Can you work these out from the model? Positions are in its coordinate system, mm. Face numbers are marked on the shaded views. Round coordinates to 2 decimals unless told otherwise and drop trailing zeros. Order: outer loops, then holes, each group sorted by start corner. A loop starts at its lowest first (then second) coordinate and runs counter-clockwise, first axis right, second up.
Q1. If we section it at A-A (z = 38): Please give me the cut outline in (x, y) (1 decimal).
Q2. If I drill on line 1 (X direction, y = 0.75, z = 38) (1 decimal); line 2 (X direction, y = 2, z = 41.5); line 3 (Z direction, x = -10, y = 2), over which ranges is the centre line in solid material (lowest first)?
Q3. If we section it at B-B (y = -2.5): Please give me the cut outline in (x, z), plus the area to 3 significant figures.
Q4. We'd pull the mould along X, two halves only. Please class the marked faces 1 and 2: pulls with the +X half, pulls with the -X half, needs draft (parallel to the pull), parting line crosses it, or undercut.
Q5. If we section it at C-C (x = 30): Please give me the cut outline in (y, z) (3 decimals).
Q6. Will these pins go through, and if not, where does the flat tip stop? P1, Ø3.5, axis at x = -30.5, y = 2.5, coming from the +Z side; P2, Ø2.5, axis at x = 24.5, y = 1.5, coming from the +Z side.
Q7. If we section it at D-D (z = -5.5): Please give me the cut outline in (x, y) (1 decimal), plus the area to 3 significant figures.
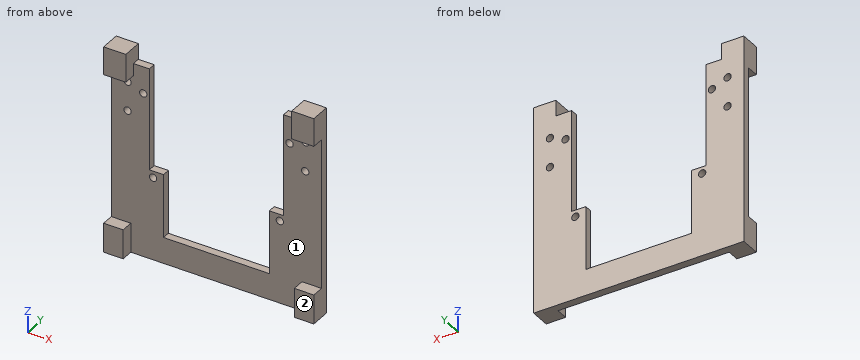
from build123d import *

# Parameters (mm, degrees)
BOSS_EXTRUDE4_DEPTH  = 3.175
M3_CLEARANCE_HOLE3_D = 3
M3_CLEARANCE_HOLE1_D = 3.1
M3_CLEARANCE_HOLE4_D = 2.95
M3_CLEARANCE_HOLE2_D = 3.1
CUT_EXTRUDE1_DEPTH   = 121.250075364
BOSS_EXTRUDE6_DEPTH  = 3.175
CUT_EXTRUDE3_DEPTH   = 121.250075364
SKETCH25_R           = 1.5
CUT_EXTRUDE4_DEPTH   = 121.250075364
SKETCH26_W           = 55
SKETCH26_H           = 60
CUT_EXTRUDE5_DEPTH   = 10
SKETCH27_OUTSIDE_W   = 217.324
SKETCH27_OUTSIDE_H   = 197.151
SKETCH27_OUTSIDE_W_2 = 86.188981544
SKETCH27_OUTSIDE_H_2 = 85
CUT_EXTRUDE6_DEPTH   = 10
SKETCH32_W           = 68
SKETCH32_H           = 11.5
CUT_EXTRUDE9_DEPTH   = 78.908304199
SKETCH33_W           = 9.094490772
SKETCH33_H           = 11.5
SKETCH33_W_2         = 8
SKETCH33_H_2         = 12
BOSS_EXTRUDE7_DEPTH  = 5
SKETCH34_W           = 6.5
SKETCH34_H           = 3.175
BOSS_EXTRUDE8_DEPTH  = 5
SKETCH35_R           = 1.5
CUT_EXTRUDE10_DEPTH  = 79.271667052
SKETCH38_W           = 18
SKETCH38_H           = 3.175
BOSS_EXTRUDE10_DEPTH = 5.8
SKETCH39_W           = 18
SKETCH39_H           = 3.175
BOSS_EXTRUDE11_DEPTH = 5.8
SKETCH37_R           = 1.5
CUT_EXTRUDE14_DEPTH  = 79.271667052
SKETCH40_W           = 43.4
SKETCH40_H           = 8
CUT_EXTRUDE15_DEPTH  = 79.271667052


with BuildPart() as part:
    # Sketch1 → Boss-Extrude4 (new body)
    with BuildSketch(Plane(origin=(0, 0, 0), x_dir=(1, 0, 0), z_dir=(0, 1, 0))):
        with BuildLine():
            Line((-62.799553621, 32.496136604), (-73.969425011, 32.691107434))
            Line((-73.969425011, 32.691107434), (-77.053684287, 35.88495141))
            ThreePointArc((-77.053684287, 35.88495141), (-84.36642289, 10.358894189), (-83.446216027, -16.178041625))
            Line((-83.446216027, -16.178041625), (-79.680911643, -13.825218315))
            Line((-79.680911643, -13.825218315), (-69.484649137, -16.179210996))
            Line((-69.484649137, -16.179210996), (-43.094490772, -58.412292655))
            Line((-43.094490772, -58.412292655), (-43.094490772, -64.826600275))
            Line((-43.094490772, -64.826600275), (-34, -64.826600275))
            Line((-34, -64.826600275), (-34, -58.55))
            Line((-34, -58.55), (34, -58.55))
            Line((34, -58.55), (34, -64.826600275))
            Line((34, -64.826600275), (43.094490772, -64.826600275))
            Line((43.094490772, -64.826600275), (43.094490772, -58.412292655))
            Line((43.094490772, -58.412292655), (69.484649137, -16.179210996))
            Line((69.484649137, -16.179210996), (79.680911643, -13.825218315))
            Line((79.680911643, -13.825218315), (83.446216027, -16.178041625))
            ThreePointArc((83.446216027, -16.178041625), (84.36642289, 10.358894189), (77.053684287, 35.88495141))
            Line((77.053684287, 35.88495141), (73.969425011, 32.691107434))
            Line((73.969425011, 32.691107434), (62.799553621, 32.496136604))
            Line((62.799553621, 32.496136604), (30.284668021, 63.895396642))
            Line((30.284668021, 63.895396642), (30.089697191, 75.065268032))
            Line((30.089697191, 75.065268032), (33.173956467, 78.259112008))
            ThreePointArc((33.173956467, 78.259112008), (0, 85), (-33.173956467, 78.259112008))
            Line((-33.173956467, 78.259112008), (-30.089697191, 75.065268032))
            Line((-30.089697191, 75.065268032), (-30.284668021, 63.895396642))
            Line((-30.284668021, 63.895396642), (-62.799553621, 32.496136604))
        make_face()
    extrude(amount=BOSS_EXTRUDE4_DEPTH)

    # M3 Clearance Hole3 (through all)
    with Locations(Plane(origin=(0, 0, 0), x_dir=(-1, 0, 0), z_dir=(0, -1, 0))):
        with Locations((36.415, -50), (36.415, -38), (-36.415, -50), (-36.415, -38)):
            Hole(M3_CLEARANCE_HOLE3_D / 2)

    # M3 Clearance Hole1 (through all)
    with Locations(Plane(origin=(0, 3.175, 0), x_dir=(1, 0, 0), z_dir=(0, 1, 0))):
        with Locations((-78.542321426, -8.49139241), (78.542321426, -8.49139241), (74.155025063, 27.240269049), (-74.155025063, 27.240269049)):
            Hole(M3_CLEARANCE_HOLE1_D / 2)

    # M3 Clearance Hole4 (through all)
    with Locations(Plane(origin=(0, 0, 0), x_dir=(-1, 0, 0), z_dir=(0, -1, 0))):
        with Locations((-67.099301622, -15.278865202), (-50.141885166, -42.416404279), (-61.062544382, 30.698137949), (-38.043670771, 52.927205804), (50.141885166, -42.416404279), (67.099301622, -15.278865202), (38.043670771, 52.927205804), (61.062544382, 30.698137949)):
            Hole(M3_CLEARANCE_HOLE4_D / 2)

    # M3 Clearance Hole2 (through all)
    with Locations(Plane(origin=(0, 3.175, 0), x_dir=(1, 0, 0), z_dir=(0, 1, 0))):
        with Locations((27, 76.497766718), (-27, 76.497766718)):
            Hole(M3_CLEARANCE_HOLE2_D / 2)

    # Sketch20 → Cut-Extrude1 (cut, through all)
    with BuildSketch(Plane(origin=(0, 3.175, 0), x_dir=(1, 0, 0), z_dir=(0, 1, 0))):
        with BuildLine():
            Line((-14.64850035, 45.5), (-14.64850035, 40.5))
            ThreePointArc((-14.64850035, 40.5), (-16.14850035, 39), (-17.64850035, 40.5))
            Line((-17.64850035, 40.5), (-17.64850035, 45.5))
            ThreePointArc((-17.64850035, 45.5), (-16.14850035, 47), (-14.64850035, 45.5))
        make_face()
        with BuildLine():
            Line((14.64850035, 45.5), (14.64850035, 40.5))
            ThreePointArc((14.64850035, 40.5), (16.14850035, 39), (17.64850035, 40.5))
            Line((17.64850035, 40.5), (17.64850035, 45.5))
            ThreePointArc((17.64850035, 45.5), (16.14850035, 47), (14.64850035, 45.5))
        make_face()
    extrude(amount=-CUT_EXTRUDE1_DEPTH, mode=Mode.SUBTRACT)

    # Sketch22 → Boss-Extrude6 (add)
    with BuildSketch(Plane(origin=(0, 3.175, 0), x_dir=(1, 0, 0), z_dir=(0, 1, 0))):
        Polygon((-30.284668021, 63.895396642), (-30.245177733, 66.157793715), (-65.061950694, 32.535626892), (-62.799553621, 32.496136604), align=None)
        Polygon((-69.484649137, -16.179210996), (-71.689396914, -15.670204865), (-43.094490772, -61.431620518), (-43.094490772, -58.412292655), align=None)
        Polygon((43.094490772, -61.431620518), (71.689396914, -15.670204865), (69.484649137, -16.179210996), (43.094490772, -58.412292655), align=None)
        Polygon((65.061950694, 32.535626892), (30.245177733, 66.157793715), (30.284668021, 63.895396642), (62.799553621, 32.496136604), align=None)
    extrude(amount=-BOSS_EXTRUDE6_DEPTH)

    # Sketch24 → Cut-Extrude3 (cut, through all)
    with BuildSketch(Plane(origin=(0, 3.175, 0), x_dir=(1, 0, 0), z_dir=(0, 1, 0))):
        Polygon((-27, -52.75), (-27, -22.75), (-21.2, -22.75), (-21.2, 1.45), (0, 1.45), (21.2, 1.45), (21.2, -22.75), (27, -22.75), (27, -52.75), (21.2, -52.75), (21.2, -58.55), (-21.2, -58.55), (-21.2, -52.75), align=None)
    extrude(amount=-CUT_EXTRUDE3_DEPTH, mode=Mode.SUBTRACT)

    # Sketch25 → Cut-Extrude4 (cut, through all)
    with BuildSketch(Plane(origin=(0, 3.175, 0), x_dir=(1, 0, 0), z_dir=(0, 1, 0))):
        with Locations(Location((-24.1, -55.65, 0), (0, 0, 270))):
            Circle(SKETCH25_R)
        with Locations(Location((-24.1, -19.85, 0), (0, 0, 270))):
            Circle(SKETCH25_R)
        with Locations(Location((24.1, -19.85, 0), (0, 0, 270))):
            Circle(SKETCH25_R)
        with Locations(Location((24.1, -55.65, 0), (0, 0, 270))):
            Circle(SKETCH25_R)
    extrude(amount=-CUT_EXTRUDE4_DEPTH, mode=Mode.SUBTRACT)

    # Sketch26 → Cut-Extrude5 (cut)
    with BuildSketch(Plane(origin=(0, 3.175, 0), x_dir=(1, 0, 0), z_dir=(0, 1, 0))):
        with Locations((0, -28.55)):
            Rectangle(SKETCH26_W, SKETCH26_H)
    extrude(amount=-CUT_EXTRUDE5_DEPTH, mode=Mode.SUBTRACT)

    # Sketch27 outside → Cut-Extrude6 (cut)
    with BuildSketch(Plane(origin=(0, 3.175, 0), x_dir=(1, 0, 0), z_dir=(0, 1, 0))):
        with Locations((0, 10.0865)):
            Rectangle(SKETCH27_OUTSIDE_W, SKETCH27_OUTSIDE_H)
        with Locations((0, -22.326600275)):
            Rectangle(SKETCH27_OUTSIDE_W_2, SKETCH27_OUTSIDE_H_2, mode=Mode.SUBTRACT)
    extrude(amount=-CUT_EXTRUDE6_DEPTH, mode=Mode.SUBTRACT)

    # Sketch32 → Cut-Extrude9 (cut, through all)
    with BuildSketch(Plane(origin=(0, 3.175, 0), x_dir=(1, 0, 0), z_dir=(0, 1, 0))):
        with Locations((0, -59.076600275)):
            Rectangle(SKETCH32_W, SKETCH32_H)
    extrude(amount=-CUT_EXTRUDE9_DEPTH, mode=Mode.SUBTRACT)

    # Sketch33 → Boss-Extrude7 (add)
    with BuildSketch(Plane.XZ):
        with Locations((-38.547245386, 59.076600275)):
            Rectangle(SKETCH33_W, SKETCH33_H)
        with Locations((38.547245386, 59.076600275)):
            Rectangle(SKETCH33_W, SKETCH33_H)
        with Locations((-39.094490772, -14.173399725)):
            Rectangle(SKETCH33_W_2, SKETCH33_H_2)
        with Locations((39.094490772, -14.173399725)):
            Rectangle(SKETCH33_W_2, SKETCH33_H_2)
    extrude(amount=BOSS_EXTRUDE7_DEPTH)

    # Sketch34 → Boss-Extrude8 (add)
    with BuildSketch(Plane.XY.offset(53.326600275)):
        with Locations((-30.75, 1.5875)):
            Rectangle(SKETCH34_W, SKETCH34_H)
        with Locations((30.75, 1.5875)):
            Rectangle(SKETCH34_W, SKETCH34_H)
    extrude(amount=BOSS_EXTRUDE8_DEPTH)

    # Sketch35 → Cut-Extrude10 (cut, through all)
    with BuildSketch(Plane(origin=(0, 3.175, 0), x_dir=(1, 0, 0), z_dir=(0, 1, 0))):
        with Locations(Location((-30, -47.326600275, 0), (0, 0, 270))):
            Circle(SKETCH35_R)
        with Locations(Location((30, -47.326600275, 0), (0, 0, 270))):
            Circle(SKETCH35_R)
    extrude(amount=-CUT_EXTRUDE10_DEPTH, mode=Mode.SUBTRACT)

    # Sketch38 → Boss-Extrude10 (add)
    with BuildSketch(Plane(origin=(-27.5, 0, 0), x_dir=(0, 0, -1), z_dir=(1, 0, 0))):
        with Locations((-7.55, 1.5875)):
            Rectangle(SKETCH38_W, SKETCH38_H)
    extrude(amount=BOSS_EXTRUDE10_DEPTH)

    # Sketch39 → Boss-Extrude11 (add)
    with BuildSketch(Plane.ZY.offset(-27.5)):
        with Locations((7.55, 1.5875)):
            Rectangle(SKETCH39_W, SKETCH39_H)
    extrude(amount=BOSS_EXTRUDE11_DEPTH)

    # Sketch37 → Cut-Extrude14 (cut, through all)
    with BuildSketch(Plane(origin=(0, 3.175, 0), x_dir=(1, 0, 0), z_dir=(0, 1, 0))):
        with Locations(Location((-26, -13.826600275, 0), (0, 0, 270))):
            Circle(SKETCH37_R)
        with Locations(Location((26, -13.826600275, 0), (0, 0, 270))):
            Circle(SKETCH37_R)
    extrude(amount=-CUT_EXTRUDE14_DEPTH, mode=Mode.SUBTRACT)

    # Sketch40 → Cut-Extrude15 (cut, through all)
    with BuildSketch(Plane(origin=(0, 3.175, 0), x_dir=(1, 0, 0), z_dir=(0, 1, 0))):
        with Locations((0, 5.45)):
            Rectangle(SKETCH40_W, SKETCH40_H)
    extrude(amount=-CUT_EXTRUDE15_DEPTH, mode=Mode.SUBTRACT)


solid = part.part
Solution:
1. outline: (-43.1, 0) - (-37.9, 0) - (-37.9, 3.2) - (-43.1, 3.2) - close; (-34.9, 0) - (-27.5, 0) - (-27.5, 3.2) - (-34.9, 3.2) - close; (27.5, 0) - (34.9, 0) - (34.9, 3.2) - (27.5, 3.2) - close; (37.9, 0) - (43.1, 0) - (43.1, 3.2) - (37.9, 3.2) - close
2. line 1: x = -43.1 to -37.9, -34.9 to -27.5, 27.5 to 34.9, 37.9 to 43.1
2. line 2: x = -43.09 to -27.5, 27.5 to 43.09
2. line 3: z = -20.17 to -9.45
3. outline: (-43.09, -20.17) - (-35.09, -20.17) - (-35.09, -8.17) - (-43.09, -8.17) - close; (-43.09, 53.33) - (-34, 53.33) - (-34, 64.83) - (-43.09, 64.83) - close; (34, 53.33) - (43.09, 53.33) - (43.09, 64.83) - (34, 64.83) - close; (35.09, -20.17) - (43.09, -20.17) - (43.09, -8.17) - (35.09, -8.17) - close
3. area: 401 mm2
4. face 1: undercut
4. face 2: needs draft
5. outline: (0, -20.173) - (3.175, -20.173) - (3.175, 45.827) - (0, 45.827) - close; (0, 48.827) - (3.175, 48.827) - (3.175, 58.327) - (0, 58.327) - close
6. P1: stops at z = 58.33
6. P2: stops at z = 16.55
7. outline: (-43.1, 0) - (-21.7, 0) - (-21.7, 3.2) - (-43.1, 3.2) - close; (21.7, 0) - (43.1, 0) - (43.1, 3.2) - (21.7, 3.2) - close
7. area: 136 mm2
